Autodesk Inventor part; units mm, degrees
ref_plane "YZ Plane" through (0, 0, 0) normal (1, 0, 0) x (0, 1, 0)
ref_plane "XZ Plane" through (0, 0, 0) normal (0, 1, 0) x (-1, 0, 0)
ref_plane "XY Plane" through (0, 0, 0) normal (0, 0, 1) x (1, 0, 0)
sketch "Sketch1" plane through (0, 0, 0) normal (0, 1, 0) x (-1, 0, 0)
  line L0 (0, 0) -> (33, 0)
  line L1 (33, 0) -> (33, -28)
  line L2 (33, -28) -> (0, -28)
  line L3 (0, -28) -> (0, 0)
  line L4 (0, -17.5) -> (-20, -17.5)
  line L5 (-20, -17.5) -> (-20, -10.5)
  line L6 (-20, -10.5) -> (0, -10.5)
  line L7 (0, -10.5) -> (0, -17.5)
  line L8 (33, -17.5) -> (53, -17.5)
  line L9 (53, -17.5) -> (53, -10.5)
  line L10 (53, -10.5) -> (33, -10.5)
  line L11 (33, -10.5) -> (33, -17.5)
  line L12 (20, -28) -> (13, -28)
  line L13 (13, -28) -> (13, -48)
  line L14 (13, -48) -> (20, -48)
  line L15 (20, -48) -> (20, -28)
  line L16 (20, 0) -> (13, 0)
  line L17 (13, 0) -> (13, 20)
  line L18 (13, 20) -> (20, 20)
  line L19 (20, 20) -> (20, 0)
  circle A0 centre (16.5, -44) radius 1.75
  circle A1 centre (-16, -14) radius 1.75
  circle A2 centre (16.5, 16) radius 1.75
  circle A3 centre (49, -14) radius 1.75
  line L20 (16.5, -44) -> (16.5, -48) construction
  line L21 (-16, -14) -> (-20, -14) construction
  line L22 (16.5, 16) -> (16.5, 20) construction
  line L23 (49, -14) -> (53, -14) construction
  circle A4 centre (43, -14) radius 1.75
  circle A5 centre (37, -14) radius 1.75
  circle A6 centre (16.5, -38) radius 1.75
  circle A7 centre (16.5, -32) radius 1.75
  circle A8 centre (-10, -14) radius 1.75
  circle A9 centre (-4, -14) radius 1.75
  circle A10 centre (16.5, 10) radius 1.75
  circle A11 centre (16.5, 4) radius 1.75
  point P0 (16.5, -28)
  point P1 (16.5, 0)
  point P2 (0, -14)
  point P3 (33, -14)
  dimension "d0" = 33
  dimension "d1" = 28
  dimension "d29" = 7
  dimension "d34" = 20
  dimension "d35" = 4
  dimension "d36" = 3.5
  dimension "d44" = 6
  dimension "d51" = 6
  dimension "d58" = 6
  dimension "d65" = 6
extrude "Extrusion1" add sketch "Sketch1" along normal blind 2
sketch "Sketch2" plane through (0, 2, 0) normal (0, 1, 0) x (1, 0, 0)
  line L0 (0, 28) -> (-13, 28)
  line L1 (-33, 28) -> (-33, 17.5)
  line L2 (-33, 0) -> (-20, 0)
  line L3 (0, 0) -> (0, 10.5)
  line L4 (-26.6, 1.85) -> (-6.4, 1.85)
  line L5 (-6.4, 1.85) -> (-6.4, 4.05)
  line L6 (-6.4, 4.05) -> (-26.6, 4.05)
  line L7 (-26.6, 4.05) -> (-26.6, 1.85)
  line L8 (-26.6, 23.95) -> (-6.4, 23.95)
  line L9 (-6.4, 23.95) -> (-6.4, 26.15)
  line L10 (-6.4, 26.15) -> (-26.6, 26.15)
  line L11 (-26.6, 26.15) -> (-26.6, 23.95)
  line L12 (-26.6, 1.85) -> (-33, 1.85)
  line L13 (-26.6, 1.85) -> (-26.6, 0)
  line L14 (-26.6, 26.15) -> (-26.6, 28)
  line L15 (-6.4, 4.05) -> (0, 4.05)
  line L16 (-13, 28) -> (-13, 48)
  line L17 (-13, 48) -> (-20, 48)
  line L18 (-20, 48) -> (-20, 28)
  line L19 (-20, 28) -> (-33, 28)
  line L20 (-33, 17.5) -> (-53, 17.5)
  line L21 (-53, 17.5) -> (-53, 10.5)
  line L22 (-53, 10.5) -> (-33, 10.5)
  line L23 (-33, 10.5) -> (-33, 0)
  line L24 (-20, 0) -> (-20, -20)
  line L25 (-20, -20) -> (-13, -20)
  line L26 (-13, -20) -> (-13, 0)
  line L27 (-13, 0) -> (0, 0)
  line L28 (0, 10.5) -> (20, 10.5)
  line L29 (20, 10.5) -> (20, 17.5)
  line L30 (20, 17.5) -> (0, 17.5)
  line L31 (0, 17.5) -> (0, 28)
  line L32 (-28.5, 21.5) -> (-4.5, 21.5)
  line L33 (-4.5, 21.5) -> (-4.5, 6.5)
  line L34 (-4.5, 6.5) -> (-28.5, 6.5)
  line L35 (-28.5, 6.5) -> (-28.5, 21.5)
  line L36 (-28.5, 21.5) -> (-4.5, 6.5) construction
  line L37 (-4.5, 21.5) -> (-28.5, 6.5) construction
  point P0 (-16.5, 14)
  point P1 (-16.5, 23.95)
  point P2 (20, 14)
  dimension "d4" = 2.2
  dimension "d5" = 20.2
  dimension "d6" = 19.9
  dimension "d37" = 24
  dimension "d38" = 15
extrude "Extrusion2" cut sketch "Sketch2" against normal through all contours L10 L9 L8 L11 | L5 L4 L7 L6 | L32 L33 L34 L35
fillet "Fillet1" radius 3.5 8 edges at (-20, 1, 20) (-13, 1, 20) (20, 1, -10.5) (20, 1, -17.5) (-13, 1, -48) (-20, 1, -48) (-53, 1, -17.5) (-53, 1, -10.5)
fillet "Fillet2" radius 7 4 edges at (-33, 1, 0) (-33, 1, -28) (0, 1, -28) (0, 1, 0)
fillet "Fillet3" radius 2 4 edges at (-28.5, 1, -21.5) (-4.5, 1, -21.5) (-28.5, 1, -6.5) (-4.5, 1, -6.5)
sketch "Sketch4" plane through (0, 2, 0) normal (0, 1, 0) x (1, 0, 0)
  arc A0 (-4.5, 19.5) -> (-6.5, 21.5) centre (-6.5, 19.5) ccw construction
  line L0 (-26.5, 21.5) -> (-6.5, 21.5) construction
  line L1 (-4.5, 19.5) -> (-4.5, 8.5) construction
  arc A1 (-6.5, 6.5) -> (-4.5, 8.5) centre (-6.5, 8.5) ccw construction
  line L2 (-6.5, 6.5) -> (-26.5, 6.5) construction
  arc A2 (-28.5, 8.5) -> (-26.5, 6.5) centre (-26.5, 8.5) ccw construction
  line L3 (-28.5, 8.5) -> (-28.5, 19.5) construction
  arc A3 (-26.5, 21.5) -> (-28.5, 19.5) centre (-26.5, 19.5) ccw construction
  line L4 (-25.5, 21.5) -> (-23.5, 21.5)
  line L5 (-23.5, 21.5) -> (-23.5, 6.5)
  line L6 (-23.5, 6.5) -> (-25.5, 6.5)
  line L7 (-25.5, 6.5) -> (-25.5, 21.5)
  line L8 (-9.5, 6.5) -> (-7.5, 6.5)
  line L9 (-7.5, 6.5) -> (-7.5, 21.5)
  line L10 (-7.5, 21.5) -> (-9.5, 21.5)
  line L11 (-9.5, 21.5) -> (-9.5, 6.5)
  point P0 (0, 0)
  dimension "d70" = 3
  dimension "d71" = 3
  dimension "d72" = 2
extrude "Extrusion4" add sketch "Sketch4" against normal up to surface (2 mm away)
properties part number "SoporteMarkers12"
Geometry: final body of the model. Coordinates: model frame, mm. A direction names the side the tool comes from. Round coordinates to 2 decimals unless told otherwise and drop trailing zeros. Order: outer loops, then holes, each group sorted by start corner. A loop starts at its lowest first (then second) coordinate and runs counter-clockwise, first axis right, second up. Notation, with made-up numbers: (11, -29.5) -> (54, -29.5) arc R29 cw to (54, -7.5) -> close; hole circle Ø7 at (22, 63). An arc over 180 degrees is marked (long way). Use one line per item in the form item = value.
(1) First-contact query: pin 1 Ø0.8 at (x, y) = (-7, 1) entering from +Z; pin 2 Ø1 at (x, y) = (-15.5, 1) entering from +Z; pin 3 Ø0.5 at (x, y) = (-7, 1) entering from -Z. Flat tips, straight axial feed; report the tip coordinate or a pass-through.
Results list:
pin_1 = 0
pin_2 = 19.96
pin_3 = -28
(2) Section B-B on z = -32. Return loops of the section in (x, y).
Results list:
outline = (-20, 0) -> (-18.25, 0) -> (-18.25, 2) -> (-20, 2) -> close; (-14.75, 0) -> (-13, 0) -> (-13, 2) -> (-14.75, 2) -> close
(3) Section C-C on y = 1.1. Count the separate pieces of the cut face and the enclosed holes in it, and give its area (3 significant figures).
Results list:
separate_pieces = 1
enclosed_holes = 17
area = 920 mm^2
(4) Ray query, probe 1 along Z at (x, y) = (-6.5, 0.3); probe 2 along Z at (x, y) = (-37, 0.95); probe 3 along Z at (x, y) = (-14.5, 1.45). Return the intervals inside material, ascending. Write a range as [from, to].
Results list:
probe_1 = [-27.98, -26.15], [-23.95, -21.5], [-6.5, -4.05], [-1.85, -0.02]
probe_2 = [-17.5, -15.75], [-12.25, -10.5]
probe_3 = [-47.37, -26.15], [-23.95, -21.5], [-6.5, -4.05], [-1.85, 19.37]
(5) Section A-A on x = 4. Return loops of the section in (y, z).
Results list:
outline = (0, -17.5) -> (2, -17.5) -> (2, -15.75) -> (0, -15.75) -> close; (0, -12.25) -> (2, -12.25) -> (2, -10.5) -> (0, -10.5) -> close
(6) Access query for faces 1 (the face through (-26.6, 1, -25)), 2 (the face through (-10, 1, -28)). Directions: +Z, -Z, +X, -X, +Y, -Y. A direction counts if a zero-diameter tool reaches every point of the face in a straight line with its end or side. Return the directions, or none.
Results list:
face_1 = +Y, -Y
face_2 = -Z, +X, +Y, -Y
(7) Section D-D on x = -40. Return loops of the section in (y, z), and give its area (3 significant figures).
Results list:
outline = (0, -17.5) -> (2, -17.5) -> (2, -10.5) -> (0, -10.5) -> close
area = 14.0 mm^2
(8) Draft query along Z for faces 3 (the face through (16.228, 0.986, -15.735)), 4 (the face through (-2, 1, -25.9)), 5 (the face through (-41, 1, -10.5)). Return one class per face: pulls with the +Z half, pulls with the -Z half, needs draft (parallel to the pull), parting line crosses it, or undercut.
Results list:
face_3 = undercut
face_4 = pulls with the -Z half
face_5 = pulls with the +Z half
